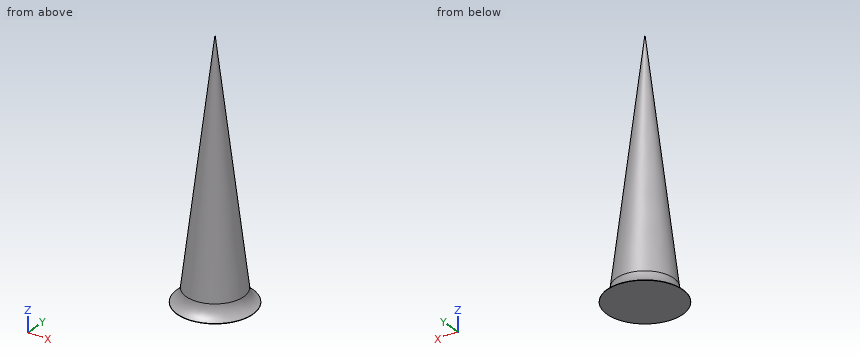
```python
from build123d import *

# Parameters (mm, degrees)
F0_R     = 85
F2_R     = 0.5
F4_R     = 105.9677495378
F5_DEPTH = 1


# Not quite as in the source:
# - a fillet or chamfer that OpenCascade refuses, or shapes differently, is made with other operations: its cross-section is extruded or revolved along the edge and cut away or added


with BuildPart() as f3:
    # F0 (on Top) → F3 section 0
    with BuildSketch(Plane.XY):
        Circle(F0_R)
    # F2 (on offset) → F3 section 1
    with BuildSketch(Plane.XY.offset(700)):
        Circle(F2_R)
    loft()

    # F4 (on Top) → F5 (join)
    with BuildSketch(Plane.XY):
        Circle(F4_R)
    extrude(amount=F5_DEPTH)

    # F6: fillet of radius 50 on 1 edges, made by hand


with BuildPart() as f6_tool2:
    # F6_s3 → F6_t4 (revolve)
    with BuildSketch(Plane.XZ):
        with BuildLine():
            ThreePointArc((105.9675577084, 0.9996489993), (88.5489126941, 16.8340527655), (80.3057755127, 38.8837290936))
            Line((80.3057755127, 38.8837290936), (75.3416542323, 38.284488739))
            ThreePointArc((75.3416542323, 38.284488739), (77.6286078916, 19.3426481611), (79.9151644339, 0.4007596454))
            Line((79.9151644339, 0.4007596454), (84.8792857143, -4.0001589064))
            ThreePointArc((84.8792857143, -4.0001589064), (95.4234217114, -4.0001589064), (103.5696146476, -3.3879993647))
            Line((103.5696146476, -3.3879993647), (105.9675577084, 0.9996489993))
        make_face()
    revolve(axis=Axis((0, 0, 1), (0, 0, 1)))

    split(bisect_by=Plane.XY, keep=Keep.TOP)


with BuildPart() as f3_1:
    add(f3.part)

    # F6_t1: union F6_tool2
    add(f6_tool2.part)


solid = f3_1.part
```
Design review of the part built by this model. Coordinates are the model's own, in mm. Round coordinates to 2 decimals unless told otherwise and drop trailing zeros. Write each loop counter-clockwise with the first axis right and the second up, starting at its lowest first coordinate (ties: lowest second). Pieces come first, ordered by that corner, then holes.
Item 1: For probe 1 along Z at (x, y) = (95, 45.5); probe 2 along Z at (x, y) = (19, 89); probe 3 along Y at (x, z) = (48, 208.5), list the stretches that pass through material, from the lowest coordinate up.
Item 2: Clearance check with flat-ended pins moving along their axes: pin 1 Ø5 at (y, z) = (-26, 70.5) entering from +X; pin 2 Ø5 at (x, z) = (33, 297) entering from +Y; pin 3 Ø1.5 at (y, z) = (23.5, 356) entering from -X; pin 4 Ø12 at (x, y) = (-70.5, -5) entering from -Z. State where each tip first meets the part, or that it passes through.
Item 3: We need section A-A on z = 400. Write out the cut boundary in (x, y).
Item 4: We need section B-B on z = 147. Write out the cut boundary in (x, y) (3 decimals), and give its area (3 significant figures).
Returned:
1. probe 1: z = 0 to 1.35
1. probe 2: z = 0 to 13.51
1. probe 3: y = -35.72 to 35.72
2. pin 1: stops at x = 72.85
2. pin 2: stops at y = 38.58
2. pin 3: stops at x = -35.35
2. pin 4: stops at z = 0
3. outline: circle Ø73.43 at (0, 0)
4. outline: circle Ø134.51 at (0, 0)
4. area: 14,200 mm2
